Could you check a few things on this drawing? It's one solid part, dimensions in mm from its lowest x, y, z. A direction names the side the tool comes from. Give positions to 0.01 mm unless a question says otherwise; leave off trailing zeros. Loops run counter-clockwise (first coordinate to the right, second up) from the corner with the lowest first, then second, coordinate; pieces in that order, holes last. Notation, with made-up numbers: M 55,73 L 75,73 A14 ccw 75,90 Z; hole C -15,6.5 d11. An arc over 180 degrees is marked long. Answer as a JSON object with one key per item and string values.
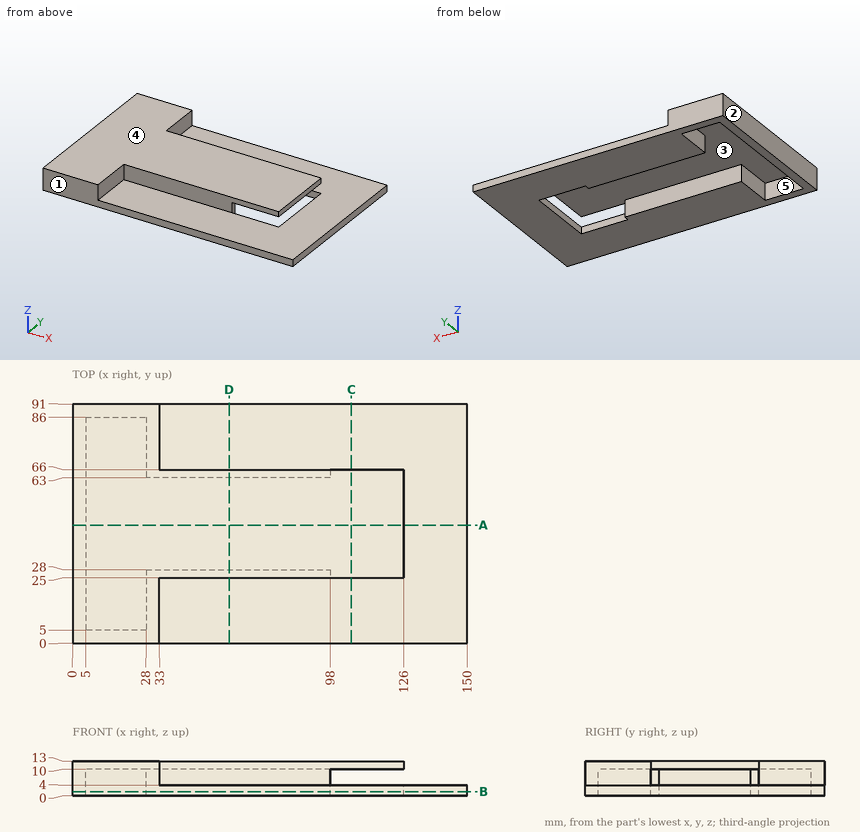
1) Suppose I cut it at B-B, the plane z = 1.5. Write out the boundary of the cut face in (x, y).
Answer list:
{"outline": "M 0,0 L 150,0 L 150,91 L 0,91 Z; hole M 5,5 L 28,5 L 28,28 L 98,28 L 98,25 L 126,25 L 126,66 L 98,66 L 98,63 L 28,63 L 28,86 L 5,86 Z"}
2) Please list where these lines run through material, in increasing order: line 1 along X through (y, z) = (12, 6.25); line 2 along Y through (x, z) = (53, 8); line 3 along X through (y, z) = (40.5, 1). Write a range as from..to.
Answer list:
{"line 1": "0..5, 28..33", "line 2": "25..28, 63..66", "line 3": "0..5, 126..150"}
3) Suppose I cut it at A-A, the plane y = 45. Write out the boundary of the cut face in (x, z).
Answer list:
{"outline": "M 0,0 L 5,0 L 5,10 L 126,10 L 126,13 L 0,13 Z; M 126,0 L 150,0 L 150,4 L 126,4 Z"}
4) If we mould it in two halves opening along X, with no side actions, what happens to the marked faces 1, 2 and 3? For each: +X half, -X half, draft (parallel to the pull), parting line (faces both ways), or undercut.
Answer list:
{"face 1": "draft", "face 2": "-X half", "face 3": "undercut"}
5) Suppose I cut it at C-C, the plane x = 106. Write out the boundary of the cut face in (y, z).
Answer list:
{"outline": "M 0,0 L 25,0 L 25,4 L 0,4 Z; M 25,10 L 66,10 L 66,13 L 25,13 Z; M 66,0 L 91,0 L 91,4 L 66,4 Z"}
6) For the marked faces 4 and 5, which set-ups out of +Z, -Z, +X, -X, +Y, -Y let a thin tool reach every point of the face, with its end or its side?
Answer list:
{"face 4": "+Z, +X, -X, +Y, -Y", "face 5": "-Z"}
7) Will these pins go through, and if not, where does the flat tip stop? pin 1 Ø5 at (y, z) = (52, 7) entering from +X; pin 2 Ø12 at (x, y) = (26.5, 49.5) entering from -Z; pin 3 Ø4.5 at (x, z) = (87.5, 7) entering from -Y.
Answer list:
{"pin 1": "x = 5", "pin 2": "z = 10", "pin 3": "y = 25"}
8) Suppose I cut it at D-D, the plane x = 59.5. Write out the boundary of the cut face in (y, z).
Answer list:
{"outline": "M 0,0 L 28,0 L 28,10 L 63,10 L 63,0 L 91,0 L 91,4 L 66,4 L 66,13 L 25,13 L 25,4 L 0,4 Z"}
